Autodesk Fusion 360 part; units mm, degrees
sketch "Sketch1" plane through (0, 0, 0) normal (0, 0, 1) x (1, 0, 0) in component "Base"
  line L0 (-85, -115) -> (-85, 115)
  line L1 (-85, 115) -> (85, 115)
  line L2 (85, -115) -> (-85, 115) construction
  line L3 (-85, -115) -> (85, 115) construction
  line L4 (-85, -115) -> (-85, 115)
  line L5 (85, 115) -> (85, -25)
  line L6 (-85, -115) -> (5, -115)
  line L7 (85, -25) -> (5, -115)
  dimension "d1" = 170
  dimension "d2" = 230
  dimension "d3" = 140
  dimension "d4" = 90
extrude "Extrude1" add sketch "Sketch1" along normal blind 60 in component "Base"
sketch "Sketch2" plane through (0, 0, 60) normal (0, 0, 1) x (-1, 0, 0) in component "Base"
  line L0 (85, 115) -> (-5, 115)
  line L1 (-5, 115) -> (-85, 25)
  line L2 (-85, 25) -> (-85, -115)
  line L3 (-85, -115) -> (85, -115)
  line L4 (85, -115) -> (85, 115)
  line L5 (-85, -115) -> (-85, -95)
  line L6 (85, -115) -> (85, -75)
  line L7 (85, -75) -> (-65, -75)
  line L8 (-65, -75) -> (-85, -95)
  dimension "d7" = 20
  dimension "d8" = 40
  dimension "d9" = 150
extrude "Extrude2" add sketch "Sketch2" along normal blind 70 contours L2 L3 L4 L5 L6 L7 L8 in component "Base"
sketch "Sketch3" plane through (0, 0, 60) normal (0, 0, 1) x (-1, 0, 0) in component "Base"
  line L0 (-65, -75) -> (85, -75)
  line L1 (85, -75) -> (85, 115)
  line L2 (85, 115) -> (-5, 115)
  line L3 (-5, 115) -> (-85, 25)
  line L4 (-85, 25) -> (-85, -95)
  line L5 (-85, -95) -> (-65, -75)
  line L6 (85, -75) -> (85, 115)
  line L7 (85, 115) -> (65, 115)
  line L8 (65, 115) -> (65, 75)
  line L9 (85, -75) -> (5, -75)
  line L10 (5, -75) -> (5, -15)
  line L11 (5, -15) -> (65, 75)
  dimension "d12" = 20
  dimension "d13" = 40
  dimension "d14" = 80
  dimension "d15" = 60
extrude "Extrude3" add sketch "Sketch3" along normal blind 40 contours L0 L1 L2 L6 L7 L8 L9 L10 L11 in component "Base"
sketch "Sketch4" plane through (0, 75, 0) normal (0, -1, 0) x (1, 0, 0) in component "Base"
  line L0 (-5, 100) -> (-5, 60)
  line L1 (-5, 60) -> (65, 60)
  line L2 (65, 60) -> (65, 130)
  line L3 (65, 130) -> (-85, 130)
  line L4 (-85, 130) -> (-85, 100)
  line L5 (-85, 100) -> (-5, 100)
  line L6 (65, 130) -> (25, 130)
  line L7 (65, 130) -> (35, 130)
  line L8 (65, 130) -> (65, 100)
  circle A0 centre (35, 100) radius 10
  dimension "d19" = 30
extrude "Extrude4" cut sketch "Sketch4" against normal up to surface (40 mm away) contours A0 in component "Base"
sketch "Sketch5" plane through (0, 0, 100) normal (0, 0, 1) x (-1, 0, 0) in component "Base"
  line L0 (85, -75) -> (85, 115)
  line L1 (85, 115) -> (65, 115)
  line L2 (65, 115) -> (65, 75)
  line L3 (65, 75) -> (5, -15)
  line L4 (5, -15) -> (5, -75)
  line L5 (5, -75) -> (85, -75)
  line L6 (85, -75) -> (45, -75)
  line L7 (85, -75) -> (85, -45)
  circle A0 centre (45, -45) radius 10
  dimension "d22" = 30
  dimension "d23" = 20
extrude "Extrude5" cut sketch "Sketch5" against normal up to surface (100 mm away) contours A0 in component "Base"
component "Base" placed x (1, 0, 0) y (0, 1, 0) z (0, 0, 1) at (0, 0, 0)
Build history of the part. All positions in model axes, mm. A direction names the side the tool comes from. Coordinates: 2 decimals unless noted, no trailing zeros. Order: outer loops, then holes, each group sorted by start corner. A loop starts at its lowest first (then second) coordinate and runs counter-clockwise, first axis right, second up. Notation, with made-up numbers: (32, 80) - (67, 80) arc R16 cw to (67, 105) - close; hole circle Ø9 at (-1, 50.25). An arc over 180 degrees is marked (long way). Write each question's results on one line, items separated by ' | '. Start each with the question number.
Item 1: Tool access for faces 4 (the face through (-1, 115, 64)), 5 (the face through (-5, 45, 80)), 6 (the face through (-53, 0, 100)): list every direction of +Z, -Z, +X, -X, +Y, -Y with a clear straight run to the whole face (end or side of a thin tool).
Item 2: Flat gauge pins, fed straight in: pin 1 (1.5 mm diameter, centred on x = 10, z = 69, fed in from -Y); pin 2 (1.5 mm diameter, centred on y = 44.5, z = 69, fed in from +X); pin 3 (2 mm diameter, centred on x = -32.5, y = -13, fed in from +Z); pin 4 (16 mm diameter, centred on x = -45, y = 45, fed in from -Z). Where does each tip first touch, or does it go through?
Item 3: Band-saw the part on A-A on x = 35. Write the cut outline in (y, z).
Item 4: Band-saw the part on B-B on y = 45. Write the cut outline in (x, z), and give its area (3 significant figures).
Item 5: Band-saw the part on D-D on x = -10.5. Write the cut outline in (y, z).
Item 6: Wall check: probe 1 along Z at (x, y) = (35, 107); probe 2 along Y at (x, z) = (-45, 31); probe 3 along X at (y, z) = (45, 46.5). Give the ranges that are in metal, low to high. Write a range as [from, to].
Item 7: Band-saw the part on C-C on z = 18. Write the cut outline in (x, y), and give its area (3 significant figures).
Item 8: Mould opens along Y. For faces 1 (the face through (-42.83, 54.76, 50.7)), 2 (the face through (26, -9, 60)), 3 (the face through (-34.6, -29.4, 79.7)) say: released by +Y, released by -Y, zero draft, split by the parting line, or undercut.
Numbers:
1) face 4: +Z, -Z, +X, -X, +Y | face 5: +Z, +X, -Y | face 6: +Z, +X, -X, -Y
2) pin 1: y = 75 | pin 2: x = -5 | pin 3: z = 100 | pin 4: through
3) outline: (-81.25, 0) - (115, 0) - (115, 90) - (75, 90) - (75, 60) - (-81.25, 60) - close; (75, 110) - (115, 110) - (115, 130) - (75, 130) - close
4) outline: (-85, 0) - (-55, 0) - (-55, 100) - (-85, 100) - close; (-35, 0) - (85, 0) - (85, 60) - (-5, 60) - (-5, 100) - (-35, 100) - close | area: 11,400 mm^2
5) outline: (-115, 0) - (115, 0) - (115, 130) - (75, 130) - (75, 100) - (6.75, 100) - (6.75, 60) - (-115, 60) - close
6) probe 1: [0, 90], [110, 130] | probe 2: [-115, 35], [55, 115] | probe 3: [-85, -55], [-35, 85]
7) outline: (-85, -115) - (5, -115) - (85, -25) - (85, 115) - (-85, 115) - close; hole circle Ø20 at (-45, 45) | area: 35,200 mm^2
8) face 1: undercut | face 2: zero draft | face 3: released by -Y
